Can you work these out from the model? Positions are in its coordinate system, mm. Coordinates: 2 decimals unless noted, no trailing zeros. Loops run counter-clockwise (first coordinate to the right, second up) from the corner with the lowest first, then second, coordinate; pieces in that order, holes last. Notation, with made-up numbers: (85.5, 78.5) -> (107.5, 78.5) arc R11 cw to (107.5, 89.5) -> close; hole circle Ø7 at (48, 22.5). An arc over 180 degrees is marked (long way). Use one line per item in the form item = value. Start each with the question number.
(1) I'm going to push a flat-ended pin straight in: pin 1 (0.9 mm diameter, centred on x = 0.5, z = 5.5, fed in from +Y). Where does the tip first touch, or does it pass through?
(2) I need wall thicknesses on line 1 (Y direction, x = 0.75, z = 2.25); line 2 (X direction, y = 1.35, z = 1.75); line 3 (Y direction, x = 7.75, z = 2.5). Which ranges of each line are inside material? Lowest first, please. Write a range as [from, to].
(3) Imagine slicing it at A-A (z = 8.5). List the corners of the cut face in (x, y) for me, plus the area to 3 significant figures.
(4) Imagine slicing it at B-B (x = 7.25). List the corners of the cut face in (y, z) for me.
```python
from build123d import *

# Parameters (mm, degrees)
BOSS_EXTRUDE1_DEPTH = 10
CHAMFER1_SIZE       = 0.2


with BuildPart() as part:
    # Sketch1 → Boss-Extrude1 (new body)
    with BuildSketch(Plane.XY):
        Polygon((0, 0), (7.8, 0), (7.8, 1), (6.8, 1), (6.8, 1.4), (1, 1.4), (1, 1), (0, 1), align=None)
    extrude(amount=BOSS_EXTRUDE1_DEPTH)

    # Chamfer1
    chamfer1_edges = [part.edges().sort_by_distance(p)[0] for p in [
        (0, 1, 5),
        (7.8, 1, 5),
    ]]
    chamfer(chamfer1_edges, length=CHAMFER1_SIZE)


solid = part.part
```
Worked out:
q1.pin_1 = 1
q2.line_1 = [0, 1]
q2.line_2 = [1, 6.8]
q2.line_3 = [0, 0.85]
q3.outline = (0, 0) -> (7.8, 0) -> (7.8, 0.8) -> (7.6, 1) -> (6.8, 1) -> (6.8, 1.4) -> (1, 1.4) -> (1, 1) -> (0.2, 1) -> (0, 0.8) -> close
q3.area = 10.1 mm2
q4.outline = (0, 0) -> (1, 0) -> (1, 10) -> (0, 10) -> close
